Build history of the part. All positions in model axes, mm. Round coordinates to 2 decimals unless told otherwise and drop trailing zeros.
from build123d import *

# Parameters (mm, degrees)
F2_DEPTH = 18.796
F3_DEPTH = 25.4


with BuildPart() as f1:
    # F0 (on Front) → F1 (revolve)
    with BuildSketch(Plane.XZ):
        Polygon((-3.1376469415, 26.0953336054), (0, 26.0995179415), (0, 36.9026255262), (-3.1376469415, 36.9026255262), align=None)
    revolve(axis=Axis((0, 0, 11.1243847059), (0, 0, -1)))

    # F2 (cut): a face of the model
    f2_faces = [f1.faces().sort_by_distance(p)[0] for p in [
        (0, 0, 36.9026255262),
    ]]
    extrude(f2_faces, amount=-F2_DEPTH, mode=Mode.SUBTRACT)


with BuildPart() as f1b:
    # F0 (on Front) → F1, piece 2 (revolve)
    with BuildSketch(Plane.XZ):
        with BuildLine():
            Line((0, 0), (0, 16.8363694102))
            add(Edge.make_bspline(
                [(0, 16.8363694102), (-3.474241628, 12.8596777576), (-6.9484832559, 8.882986105), (-12.1888345, 6.1778346719)],
                knots=[0, 0, 0, 0, 0.2663691303, 0.2663691303, 0.2663691303, 0.2663691303], degree=3))
            add(Edge.make_bspline(
                [(-12.1888345, 6.1778346719), (-16.7755084747, 3.810121689), (-29.2204528037, 0.8901901789), (-10.2664559429, -10.2391590135), (-5.7337599776, -17.3964564632), (-3.5136023088, -20.9021689447)],
                knots=[0.2663691303, 0.2663691303, 0.2663691303, 0.2663691303, 0.4995115859, 0.7548560064, 1, 1, 1, 1], degree=3))
            Line((-3.5136023088, -20.9021689447), (-3.5625977907, -23.424660787))
            Line((-3.5625977907, -23.424660787), (-1.886081649, -23.4572245063))
            Line((-1.886081649, -23.4572245063), (0, -23.4938587097))
            Line((0, -23.4938587097), (0, -20.6523918138))
            Line((0, -20.6523918138), (0, -15.5456149951))
            Line((0, -15.5456149951), (0, -3.8507485297))
            Line((0, -3.8507485297), (0, 0))
        make_face()
        Polygon((0, -23.4938587097), (-1.886081649, -23.4572245063), (-1.886081649, -25.1011773944), (0, -25.1011773944), align=None)
    revolve(axis=Axis((0, 0, 11.1243847059), (0, 0, -1)))

    # F3 (cut): a face of the model
    f3_faces = [f1b.faces().sort_by_distance(p)[0] for p in [
        (0, 0, -25.1011773944),
    ]]
    extrude(f3_faces, amount=-F3_DEPTH, mode=Mode.SUBTRACT)


solid = f1b.part
(1) Pin check, flat tips, straight feed: P1, Ø10, axis at x = 12.5, y = -0.5, coming from the +Z side; P2, Ø4, axis at y = -4.5, z = -15, coming from the +X side; P3, Ø8, axis at y = -3.5, z = -15.5, coming from the -X side. Stop position of each tip, or through.
Responses:
P1: stops at z = 9.23
P2: stops at x = 8.4
P3: stops at x = -10.4
(2) Pull direction Z, two halves, no side cores. Call faces 1 (the face through (0.767, -3.454, -22.181)), 2 (the face through (0, 0, 0.299)), 3 (the face through (1.497, -1.148, -11.745)): +Z half, -Z half, draft (parallel to the pull), parting line (faces both ways), or undercut.
Responses:
face 1: undercut
face 2: -Z half
face 3: draft
(3) Probe line 1 (Z direction, x = -13.5, y = 13); line 2 (Z direction, x = 5, y = -6); line 3 (Y direction, x = 2, z = 1). List the from-to ranges inside material, lowest first.
Responses:
line 1: z = -5.18 to 3.31
line 2: z = -14.73 to 8.99
line 3: y = -22.41 to 22.41
